Source: CAD feature listing. Evaluate the final solid. Frame: model axes, mm. Face numbers are marked on the shaded views. Round coordinates to 2 decimals unless told otherwise and drop trailing zeros. Order: outer loops, then holes, each group sorted by start corner. A loop starts at its lowest first (then second) coordinate and runs counter-clockwise, first axis right, second up. Notation, with made-up numbers: (-24.5, 17.25) -> (27.5, 17.25) arc R34 ccw to (27.5, 50.25) -> close; hole circle Ø7 at (51, 77.5). An arc over 180 degrees is marked (long way). Use a Markdown table: item, result. Add a question column.
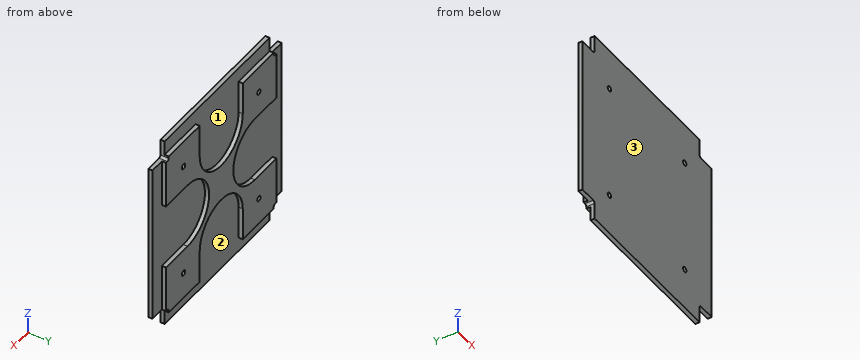
```python
from build123d import *

# Parameters (mm, degrees)
BASE_DEPTH                         = 2
ANTENNA_STORAGE_DEPTH              = 2
M3X0_5_TAPPED_HOLES_FOR_MOUNTING_D = 2.5


with BuildPart() as part:
    # Sketch1 → Base (new body)
    with BuildSketch(Plane(origin=(0, 0, 0), x_dir=(1, 0, 0), z_dir=(0, 1, 0))):
        with BuildLine():
            Line((0, 9), (8, 9))
            ThreePointArc((8, 9), (8.707106781, 8.707106781), (9, 8))
            Line((9, 8), (9, 0))
            Line((9, 0), (87, 0))
            Line((87, 0), (87, 8))
            ThreePointArc((87, 8), (87.292893219, 8.707106781), (88, 9))
            Line((88, 9), (96, 9))
            Line((96, 9), (96, 87))
            Line((96, 87), (88, 87))
            ThreePointArc((88, 87), (87.292893219, 87.292893219), (87, 88))
            Line((87, 88), (87, 96))
            Line((87, 96), (9, 96))
            Line((9, 96), (9, 88))
            ThreePointArc((9, 88), (8.707106781, 87.292893219), (8, 87))
            Line((8, 87), (0, 87))
            Line((0, 87), (0, 9))
        make_face()
    extrude(amount=BASE_DEPTH)

    # Sketch2 → Antenna Storage (add)
    with BuildSketch(Plane(origin=(0, 2, 0), x_dir=(1, 0, 0), z_dir=(0, 1, 0))):
        with BuildLine():
            Line((32, 89), (32, 73))
            ThreePointArc((32, 73), (48, 57), (64, 73))
            Line((64, 73), (64, 89))
            Line((64, 89), (87, 89))
            Line((87, 89), (87, 88))
            ThreePointArc((87, 88), (87.292893219, 87.292893219), (88, 87))
            Line((88, 87), (89, 87))
            Line((89, 87), (89, 64))
            Line((89, 64), (73, 64))
            ThreePointArc((73, 64), (57, 48), (73, 32))
            Line((73, 32), (89, 32))
            Line((89, 32), (89, 9))
            Line((89, 9), (88, 9))
            ThreePointArc((88, 9), (87.292893219, 8.707106781), (87, 8))
            Line((87, 8), (87, 7))
            Line((87, 7), (64, 7))
            Line((64, 7), (64, 23))
            ThreePointArc((64, 23), (48, 39), (32, 23))
            Line((32, 23), (32, 7))
            Line((32, 7), (9, 7))
            Line((9, 7), (9, 8))
            ThreePointArc((9, 8), (8.707106781, 8.707106781), (8, 9))
            Line((8, 9), (7, 9))
            Line((7, 9), (7, 32))
            Line((7, 32), (23, 32))
            ThreePointArc((23, 32), (39, 48), (23, 64))
            Line((23, 64), (7, 64))
            Line((7, 64), (7, 87))
            Line((7, 87), (8, 87))
            ThreePointArc((8, 87), (8.707106781, 87.292893219), (9, 88))
            Line((9, 88), (9, 89))
            Line((9, 89), (32, 89))
        make_face()
    extrude(amount=ANTENNA_STORAGE_DEPTH)

    # M3x0.5 Tapped Holes For Mounting (through all)
    with Locations(Plane(origin=(0, 4, 0), x_dir=(-1, 0, 0), z_dir=(0, 1, 0))):
        with Locations((-20, -20), (-20, -76), (-76, -20), (-76, -76)):
            Hole(M3X0_5_TAPPED_HOLES_FOR_MOUNTING_D / 2)


solid = part.part
```
1) Section B-B on x = 20. Output: boundary loops of the cut face in (y, z), then the cut area to 3 significant figures.
2) Section A-A on z = -20. Output: boundary loops of the cut face in (x, y).
3) Section D-D on z = -85.5. Output: boundary loops of the cut face in (x, y).
4) Section C-C on y = 2.8. Count the separate pieces of the cut face and the enclosed holes in it, then the cut area to 3 significant figures.
5) Draft query along X for the marked faces 1, 2 and 3. Return one class per face: pulls with the +X half, pulls with the -X half, needs draft (parallel to the pull), parting line crosses it, or undercut.
6) First-contact query: pin 1 Ø0.6 at (x, y) = (76.5, 3) entering from +Z; pin 2 Ø1 at (x, y) = (80.5, 3.5) entering from -Z; pin 3 Ø1 at (y, z) = (3.5, -12) entering from -X. Flat tips, straight axial feed; report the tip coordinate or a pass-through.
7) Line query: probe 1 along Z at (x, y) = (76, 2.45); probe 2 along X at (y, z) = (0.85, -76); probe 3 along Z at (x, y) = (76, 1.8). Output: solid intervals per line, ascending. Write a range as from..to.
Conclusion:
| question | item | result |
|---|---|---|
| 1 | outline | (0, -96) -> (2, -96) -> (2, -89) -> (4, -89) -> (4, -77.25) -> (0, -77.25) -> close; (0, -74.75) -> (4, -74.75) -> (4, -64) -> (2, -64) -> (2, -32) -> (4, -32) -> (4, -21.25) -> (0, -21.25) -> close; (0, -18.75) -> (4, -18.75) -> (4, -7) -> (2, -7) -> (2, 0) -> (0, 0) -> close |
| 1 | area | 272 mm^2 |
| 2 | outline | (0, 0) -> (18.75, 0) -> (18.75, 4) -> (7, 4) -> (7, 2) -> (0, 2) -> close; (21.25, 0) -> (74.75, 0) -> (74.75, 4) -> (64, 4) -> (64, 2) -> (32, 2) -> (32, 4) -> (21.25, 4) -> close; (77.25, 0) -> (96, 0) -> (96, 2) -> (89, 2) -> (89, 4) -> (77.25, 4) -> close |
| 3 | outline | (0, 0) -> (96, 0) -> (96, 2) -> (89, 2) -> (89, 4) -> (64, 4) -> (64, 2) -> (32, 2) -> (32, 4) -> (7, 4) -> (7, 2) -> (0, 2) -> close |
| 4 | separate pieces | 1 |
| 4 | enclosed holes | 4 |
| 4 | area | 3,030 mm^2 |
| 5 | face 1 | undercut |
| 5 | face 2 | undercut |
| 5 | face 3 | needs draft |
| 6 | pin 1 | stops at z = -7 |
| 6 | pin 2 | stops at z = -89 |
| 6 | pin 3 | stops at x = 7 |
| 7 | probe 1 | z = -89..-77.25, -74.75..-64, -32..-21.25, -18.75..-7 |
| 7 | probe 2 | x = 0..18.75, 21.25..74.75, 77.25..96 |
| 7 | probe 3 | z = -96..-77.25, -74.75..-21.25, -18.75..0 |
